Input: part model. Units: mm. Frame: model coordinates. A direction names the side the tool comes from. Coordinates: 2 decimals unless noted, no trailing zeros. Loops run counter-clockwise (first coordinate to the right, second up) from the corner with the lowest first, then second, coordinate; pieces in that order, holes last. Notation, with made-up numbers: M 48.5,-3 L 103.5,-3 A5 cw 103.5,3 Z; hole C -24,73 d4. An arc over 180 degrees is marked long. Use a Markdown table: item, result. Add a question column.
1. Section B-B on y = 1.15. Output: boundary loops of the cut face in (x, z), then the cut area to 3 significant figures.
2. Draft query along Z for faces 1 (the cylindrical face through (1.9, 1.59, -0.08)), 2 (the flat face through (2, 2.2, 1)), 3 (the cylindrical face through (-3, 1, 0)). Return one class per face: +Z half, -Z half, draft (parallel to the pull), parting line (faces both ways), or undercut.
3. Line query: L1, parallel to Z at x = 0, y = 1.25; L2, parallel to X at y = 1.45, z = -1.65. Output: solid intervals per line, ascending. Write a range as [from, to].
4. Section A-A on z = 0. Output: boundary loops of the cut face in (x, y), then the cut area to 3 significant figures.
5. Section C-C on x = 0. Output: boundary loops of the cut face in (y, z).
6. Pin query (flat end, axial travel): pin 1 (1.1 mm diameter, centred on x = 0.5, z = -0.5, fed in from +Y). Return the tip coordinate at first contact, or that it passes through.
7. Set-up query: faces 4 (the flat face through (0, 0, 0)), 5 (the flat face through (0, 1, 0)). Return all of +Z, -Z, +X, -X, +Y, -Y with unobstructed straight access to the full face (end or side cutting, diameter ignored); none if empty.
Autodesk Fusion 360 part; units mm, degrees
sketch "Sketch1" plane through (0, 0, 0) normal (0, 1, 0) x (1, 0, 0)
  circle A0 centre (0, 0) radius 1.9
  circle A1 centre (0, 0) radius 3
  dimension "d1" = 3.8
  dimension "d2" = 6
extrude "Extrude1" add sketch "Sketch1" along normal blind 3 contours A0 | A1
sketch "Sketch2" plane through (0, 3, 0) normal (0, 1, 0) x (-1, 0, 0)
  circle A0 centre (0, 0) radius 3
  circle A1 centre (0, 0) radius 1.9
  dimension "d5" = 3.8
extrude "Extrude2" cut sketch "Sketch2" against normal blind 2 contours A1
sketch "Sketch3" plane through (0, 1, 0) normal (0, 1, 0) x (-1, 0, 0)
  circle A0 centre (0, 0) radius 1.9
  circle A1 centre (0, 0) radius 2
  circle A2 centre (0, 0) radius 1.9
  dimension "d8" = 4
extrude "Extrude3" cut sketch "Sketch3" along normal blind 2.2
sketch "Sketch4" plane through (0, 1, 0) normal (0, 1, 0) x (-1, 0, 0)
  circle A0 centre (0, 0) radius 2
  circle A1 centre (0, 0) radius 2.1
  dimension "d11" = 4.2
extrude "Extrude4" cut sketch "Sketch4" along normal blind 2.8
sketch "Sketch5" plane through (0, 1, 0) normal (0, 1, 0) x (-1, 0, 0)
  circle A0 centre (0, 0) radius 2.1
  circle A1 centre (0, 0) radius 1.9
  dimension "d14" = 3.8
extrude "Extrude5" add sketch "Sketch5" along normal blind 2
sketch "Sketch6" plane through (0, 0, 0) normal (0, 0, 1) x (1, 0, 0)
  line L0 (-3.6792, 2.2002) -> (4.0444, 2.2002)
  line L1 (4.0444, 2.2002) -> (4.0444, 3.7157)
  line L2 (4.0444, 3.7157) -> (-3.2227, 3.7157)
  line L3 (-3.2227, 3.7157) -> (-3.2227, 2.2002)
extrude "Extrude6" cut sketch "Sketch6" along normal blind 4.5 and the other way blind 4.5
Answers below:
| question | item | result |
|---|---|---|
| 1 | outline | C 0,0 d6; hole C 0,0 d3.8 |
| 1 | area | 16.9 mm² |
| 2 | face 1 | undercut |
| 2 | face 2 | draft |
| 2 | face 3 | parting line |
| 3 | L1 | z = [-3, -1.9], [1.9, 3] |
| 3 | L2 | x = [-2.51, -0.94], [0.94, 2.51] |
| 4 | outline | M -3,0 L 3,0 L 3,2.2 L 1.9,2.2 L 1.9,1 L -1.9,1 L -1.9,2.2 L -3,2.2 Z |
| 4 | area | 8.64 mm² |
| 5 | outline | M 0,-3 L 2.2,-3 L 2.2,-1.9 L 1,-1.9 L 1,1.9 L 2.2,1.9 L 2.2,3 L 0,3 Z |
| 6 | pin 1 | stops at y = 1 |
| 7 | face 4 | +Z, -Z, +X, -X, -Y |
| 7 | face 5 | +Y |
